Geometry check sheet. Reference: the model listing, model coordinates, mm. Face numbers are marked on the shaded views. A direction names the side the tool comes from. Coordinates: 2 decimals unless noted, no trailing zeros. Write each loop counter-clockwise with the first axis right and the second up, starting at its lowest first coordinate (ties: lowest second). Pieces come first, ordered by that corner, then holes. Notation, with made-up numbers: (-0.75, 63) -> (37.25, 63) arc R29 ccw to (37.25, 98) -> close; hole circle Ø8 at (50, 72). An arc over 180 degrees is marked (long way). Answer in a Markdown table with one row per item. Add a question column.
1. Set-up check for the marked faces 1 and 2: record each of +Z, -Z, +X, -X, +Y, -Y from which the full face is reachable in a straight line by a thin tool's end or side.
2. Cross-section at C-C on z = -4. Record the cut outline in (x, y), and give its area (3 significant figures).
3. Mould release check, pull along Y, two halves, no side actions. Record for the marked faces 3, 4 and 5: pulls with the +Y half, pulls with the -Y half, needs draft (parallel to the pull), parting line crosses it, or undercut.
4. Cross-section at D-D on z = 0.5. Record the cut outline in (x, y).
5. Depth check by flat-ended pin: P1, Ø4, axis at y = -2, z = 1, coming from the -X side; P2, Ø1, axis at x = 2, z = 0.5, coming from the -Y side; P3, Ø1, axis at x = -3, z = -4, coming from the +Y side; P4, Ø6.5, axis at x = 0, y = 0, coming from the +Z side. Enter the tip coordinate at first touch or a pass-through.
6. Scan lines: L1, parallel to X at y = 0, z = 2.75; L2, parallel to X at y = 0, z = -1. Record each from-to range of solid material in increasing order. Write a range as from..to.
7. Cross-section at A-A on x = 0. Record the cut outline in (y, z) (3 decimals), and give its area (3 significant figures).
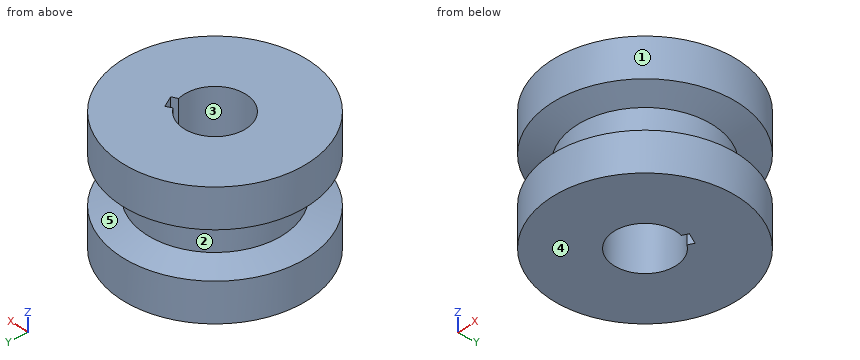
```python
from build123d import *

# Parameters (mm, degrees)
SKETCH1_R           = 7.5
SKETCH1_R_2         = 2.5
BOSS_EXTRUDE1_DEPTH = 5
CUT_EXTRUDE1_DEPTH  = 10


with BuildPart() as part:
    # Sketch1 → Boss-Extrude1 (new body, symmetric)
    with BuildSketch(Plane.XY):
        Circle(SKETCH1_R)
        Circle(SKETCH1_R_2, mode=Mode.SUBTRACT)
    extrude(amount=BOSS_EXTRUDE1_DEPTH, both=True)

    # Sketch3 → Cut-Revolve1 (revolve, cut)
    with BuildSketch(Plane(origin=(0, 0, 0), x_dir=(0, 0, -1), z_dir=(1, 0, 0))):
        Polygon((-2.5, 9.5), (-1.25, 5.5), (1.25, 5.5), (2.5, 9.5), align=None)
    revolve(axis=Axis((0, 0, 9.747557678), (0, 0, -1)), mode=Mode.SUBTRACT)

    # Sketch4 → Cut-Extrude1 (cut)
    with BuildSketch(Plane(origin=(0, 0, -5), x_dir=(-1, 0, 0), z_dir=(0, 0, -1))):
        with BuildLine():
            Line((-2.395260625, 0.716049259), (-2.835991961, 0.952176109))
            Line((-2.835991961, 0.952176109), (-2.36373826, 1.833638781))
            Line((-2.36373826, 1.833638781), (-1.923006924, 1.597511931))
            ThreePointArc((-1.923006924, 1.597511931), (-2.203656681, 1.180634251), (-2.395260625, 0.716049259))
        make_face()
    extrude(amount=-CUT_EXTRUDE1_DEPTH, mode=Mode.SUBTRACT)


solid = part.part
```
Results found:
| question | item | result |
|---|---|---|
| 1 | face 1 | +Z, -Z |
| 1 | face 2 | none |
| 2 | outline | circle Ø15 at (0, 0); hole (1.92, 1.6) arc R2.5 ccw (long way) to (2.4, 0.72) -> (2.84, 0.95) -> (2.36, 1.83) -> close |
| 2 | area | 157 mm^2 |
| 3 | face 3 | undercut |
| 3 | face 4 | needs draft |
| 3 | face 5 | parting line crosses it |
| 4 | outline | circle Ø11 at (0, 0); hole (1.92, 1.6) arc R2.5 ccw (long way) to (2.4, 0.72) -> (2.84, 0.95) -> (2.36, 1.83) -> close |
| 5 | P1 | stops at x = -7.5 |
| 5 | P2 | stops at y = -5.29 |
| 5 | P3 | stops at y = 7.07 |
| 5 | P4 | stops at z = 5 |
| 6 | L1 | x = -7.5..-2.5, 2.5..7.5 |
| 6 | L2 | x = -5.5..-2.5, 2.5..5.5 |
| 7 | outline | (-7.5, -5) -> (-2.5, -5) -> (-2.5, 5) -> (-7.5, 5) -> (-7.5, 1.875) -> (-5.5, 1.25) -> (-5.5, -1.25) -> (-7.5, -1.875) -> close; (2.5, -5) -> (7.5, -5) -> (7.5, -1.875) -> (5.5, -1.25) -> (5.5, 1.25) -> (7.5, 1.875) -> (7.5, 5) -> (2.5, 5) -> close |
| 7 | area | 87.5 mm^2 |
